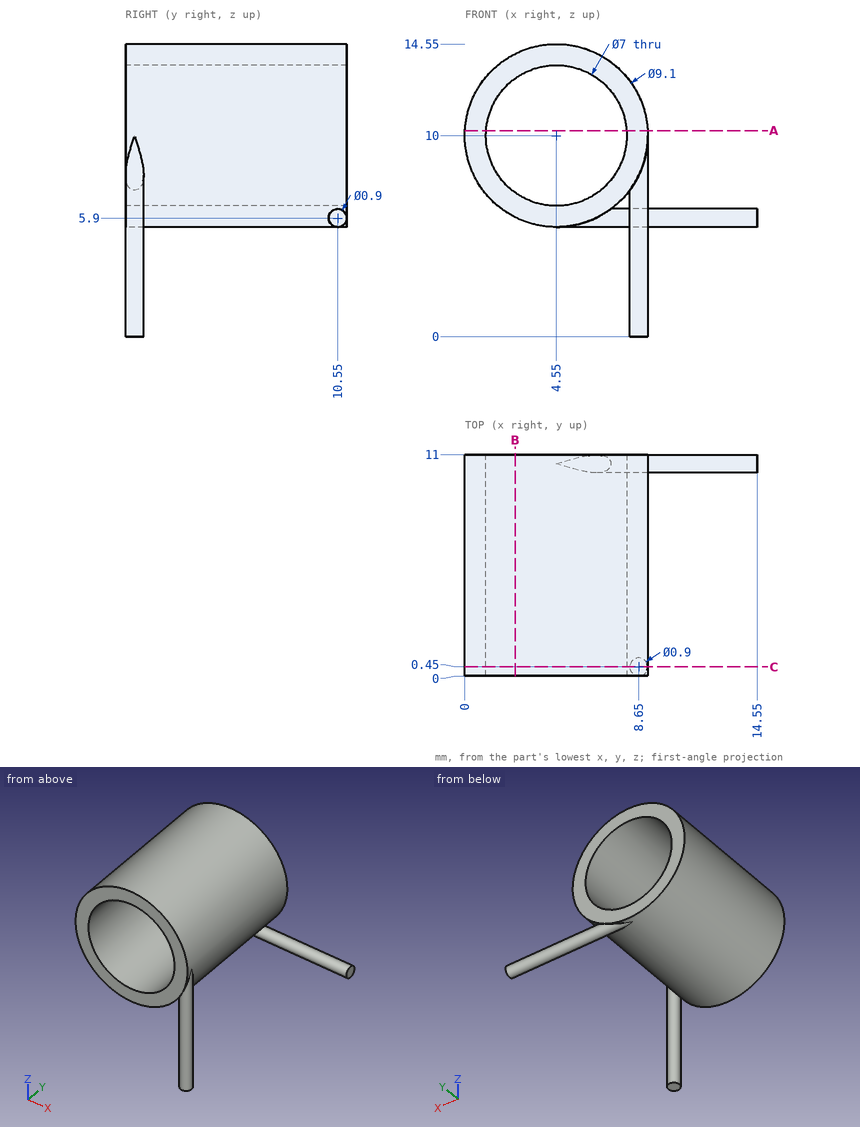
Study the drawing (mm; zero at the part's minimum x, y, z) and answer. Give positions to 0.01 mm unless a question says otherwise; leave off trailing zeros. Write each loop counter-clockwise with the first axis right and the second up, starting at its lowest first coordinate (ties: lowest second). Pieces come first, ordered by that corner, then holes. Notation, with made-up numbers: (17.5, -27) - (69.5, -27) arc R21 ccw to (69.5, 10) - close; hole circle Ø1 at (29.5, 80.5). An arc over 180 degrees is marked (long way). Use CSV: the item, a comma, the result in double quotes. Start each with the question number.
(1) Find section C-C (y = 0.45). Give the vertices of the cut face in (x, z), plus the area to 3 significant figures.
(2) Given P1, Ø1, axis at y = 6.5, z = 5.5, coming from the -X side; P2, Ø4, axis at x = 6.5, y = 8, coming from the +Z side; P3, Ø1.5, axis at y = 5, z = 5.5, coming from the +X side; P4, Ø2, axis at y = 7.5, z = 7, coming from the +X side, each flat-ended and moving along its own axis, determine where each tip first touches the part or whether it passes through.
(3) Consider line 1 along Z through (x, y) = (4.55, 3.5); line 2 along X through (y, z) = (3.5, 9); line 3 along Z through (x, y) = (2.25, 5.5). Determine where each line is inside the solid, lowest interval first.
(4) Find section A-A (z = 10.25). Give the vertices of the cut face in (x, y).
(5) Find section B-B (x = 2.5). Give the vertices of the cut face in (y, z).
Findings below:
1,outline,"(8.2, 0) - (9.1, 0) - (9.1, 10) arc R4.55 ccw (long way) to (8.2, 7.28) - close; hole circle Ø7 at (4.55, 10)"
1,area,"33.9 mm2"
2,P1,"x = 2.38"
2,P2,"z = 14.55"
2,P3,"x = 7.13"
2,P4,"x = 8.64"
3,line 1,"5.45 to 6.5, 13.5 to 14.55"
3,line 2,"0.11 to 1.2, 7.9 to 8.99"
3,line 3,"6.07 to 7.36, 12.64 to 13.93"
4,outline,"(0.01, 0) - (1.06, 0) - (1.06, 11) - (0.01, 11) - close; (8.04, 0) - (9.09, 0) - (9.09, 11) - (8.04, 11) - close"
5,outline,"(0, 5.94) - (11, 5.94) - (11, 7.16) - (0, 7.16) - close; (0, 12.84) - (11, 12.84) - (11, 14.06) - (0, 14.06) - close"
